from build123d import *

# Parameters (mm, degrees)
SKETCH1_W           = 76.2
SKETCH1_H           = 50.8
SKETCH1_R           = 2.0828
BOSS_EXTRUDE1_DEPTH = 2.032
BOSS_EXTRUDE2_DEPTH = 50.8
CUT_EXTRUDE1_DEPTH  = 9.89


with BuildPart() as part:
    # Sketch1 → Boss-Extrude1 (new body, symmetric)
    with BuildSketch(Plane(origin=(0, 0, 0), x_dir=(1, 0, 0), z_dir=(0, 1, 0))):
        Rectangle(SKETCH1_W, SKETCH1_H)
        with Locations((28.956, 19.05)):
            Circle(SKETCH1_R, mode=Mode.SUBTRACT)
        with Locations((9.144, 19.05)):
            Circle(SKETCH1_R, mode=Mode.SUBTRACT)
        with Locations((-9.144, 19.05)):
            Circle(SKETCH1_R, mode=Mode.SUBTRACT)
        with Locations((-28.956, 19.05)):
            Circle(SKETCH1_R, mode=Mode.SUBTRACT)
        Polygon((-25.4, -44.45), (25.4, -44.45), (38.1, -25.4), (-38.1, -25.4), align=None)
    extrude(amount=BOSS_EXTRUDE1_DEPTH, both=True)

    # Sketch2 → Boss-Extrude2 (add)
    with BuildSketch(Plane(origin=(0, 2.032, 0), x_dir=(1, 0, 0), z_dir=(0, 1, 0))):
        Polygon((-31.326666667, -35.56), (-25.4, -44.45), (25.4, -44.45), (31.326666667, -35.56), align=None)
    extrude(amount=BOSS_EXTRUDE2_DEPTH)

    # Sketch3 → Cut-Extrude1 (cut, through all)
    with BuildSketch(Plane(origin=(0, 0, 35.56), x_dir=(-1, 0, 0), z_dir=(0, 0, -1))):
        with BuildLine():
            ThreePointArc((-2.466199502, 25.432378782), (0, 24.257), (2.466199502, 25.432378782))
            Line((2.466199502, 25.432378782), (0, 27.432))
            Line((0, 27.432), (-2.466199502, 25.432378782))
        make_face()
        with BuildLine():
            Line((0, 27.432), (2.466199502, 25.432378782))
            ThreePointArc((2.466199502, 25.432378782), (2.992558138, 26.371235752), (3.175, 27.432))
            ThreePointArc((3.175, 27.432), (2.992558138, 28.492764248), (2.466199502, 29.431621218))
            Line((2.466199502, 29.431621218), (0, 27.432))
        make_face()
        with BuildLine():
            Line((-2.466199502, 25.432378782), (0, 27.432))
            Line((0, 27.432), (-2.466199502, 29.431621218))
            ThreePointArc((-2.466199502, 29.431621218), (-3.175, 27.432), (-2.466199502, 25.432378782))
        make_face()
        with BuildLine():
            Line((-2.466199502, 29.431621218), (0, 27.432))
            Line((0, 27.432), (2.466199502, 29.431621218))
            ThreePointArc((2.466199502, 29.431621218), (0, 30.607), (-2.466199502, 29.431621218))
        make_face()
    extrude(amount=-CUT_EXTRUDE1_DEPTH, mode=Mode.SUBTRACT)


solid = part.part
Model file for the job. Use its own axes, mm. A direction names the side the tool comes from. Give positions to 0.01 mm unless a question says otherwise; leave off trailing zeros. Loops run counter-clockwise (first coordinate to the right, second up) from the corner with the lowest first, then second, coordinate; pieces in that order, holes last. Notation, with made-up numbers: (-27, 4.5) -> (-14, 4.5) arc R13 ccw to (-14, 12.5) -> close; hole circle Ø3 at (-0.5, -22). An arc over 180 degrees is marked (long way). Use a Markdown table: item, result. Add a question column.
(1) Slice it at B-B on x = 30. List the corners of the cut face in (y, z), and give its area (3 significant figures).
(2) Tool access for faces 1 (the flat face through (-1, 2.032, 5)), 2 (the flat face through (-1, -2.032, 9)): list every direction of +Z, -Z, +X, -X, +Y, -Y with a clear straight run to the whole face (end or side of a thin tool).
(3) Slice it at A-A on z = -19.05. List the corners of the cut face in (x, y).
(4) Mould opens along X. For faces 3 (the flat face through (5, 25, 44.45)), 4 (the cylindrical face through (-26.97, -0.03, -19.68)), 5 (the flat face through (-38.1, 0, 0)) say: +X half, -X half, draft (parallel to the pull), parting line (faces both ways), or undercut.
(5) Drop flat-ended pins along their axis: pin 1 Ø3.5 at (x, z) = (28.956, -19.05) entering from -Y; pin 2 Ø8 at (x, y) = (23, 6.5) entering from -Z; pin 3 Ø12 at (x, z) = (-24.5, 12) entering from +Y; pin 4 Ø5 at (y, z) = (6, 36.5) entering from -X. Give the stop position or say it passes through.
(6) Slice it at C-C on z = 39.5. List the corners of the cut face in (x, y) (3 decimals), and give its area (3 significant figures).
(7) Slice it at D-D on y = 14. List the corners of the cut face in (x, z), and give its area (3 significant figures).
(8) Wall check: line 1 along X through (y, z) = (-1, -19); line 2 along Y through (x, z) = (-9.5, -6); line 3 along Z through (x, y) = (-14.5, 12). Give the ranges that are in metal, low to high.
Filled sheet:
| question | item | result |
|---|---|---|
| 1 | outline | (-2.03, -25.4) -> (2.03, -25.4) -> (2.03, -20.85) -> (-2.03, -20.85) -> close; (-2.03, -17.25) -> (2.03, -17.25) -> (2.03, 35.56) -> (52.83, 35.56) -> (52.83, 37.55) -> (-2.03, 37.55) -> close |
| 1 | area | 342 mm2 |
| 2 | face 1 | -Z, +X, -X, +Y |
| 2 | face 2 | +Z, -Z, +X, -X, -Y |
| 3 | outline | (-38.1, -2.03) -> (-31.04, -2.03) -> (-31.04, 2.03) -> (-38.1, 2.03) -> close; (-26.87, -2.03) -> (-11.23, -2.03) -> (-11.23, 2.03) -> (-26.87, 2.03) -> close; (-7.06, -2.03) -> (7.06, -2.03) -> (7.06, 2.03) -> (-7.06, 2.03) -> close; (11.23, -2.03) -> (26.87, -2.03) -> (26.87, 2.03) -> (11.23, 2.03) -> close; (31.04, -2.03) -> (38.1, -2.03) -> (38.1, 2.03) -> (31.04, 2.03) -> close |
| 4 | face 3 | draft |
| 4 | face 4 | undercut |
| 4 | face 5 | -X half |
| 5 | pin 1 | through |
| 5 | pin 2 | z = 35.56 |
| 5 | pin 3 | y = 2.03 |
| 5 | pin 4 | x = -31.33 |
| 6 | outline | (-28.7, -2.032) -> (28.7, -2.032) -> (28.7, 52.832) -> (-28.7, 52.832) -> close; hole circle Ø6.35 at (0, 27.432) |
| 6 | area | 3,120 mm2 |
| 7 | outline | (-31.33, 35.56) -> (31.33, 35.56) -> (25.4, 44.45) -> (-25.4, 44.45) -> close |
| 7 | area | 504 mm2 |
| 8 | line 1 | -38.1 to -31.04, -26.87 to -11.23, -7.06 to 7.06, 11.23 to 26.87, 31.04 to 38.1 |
| 8 | line 2 | -2.03 to 2.03 |
| 8 | line 3 | 35.56 to 44.45 |
